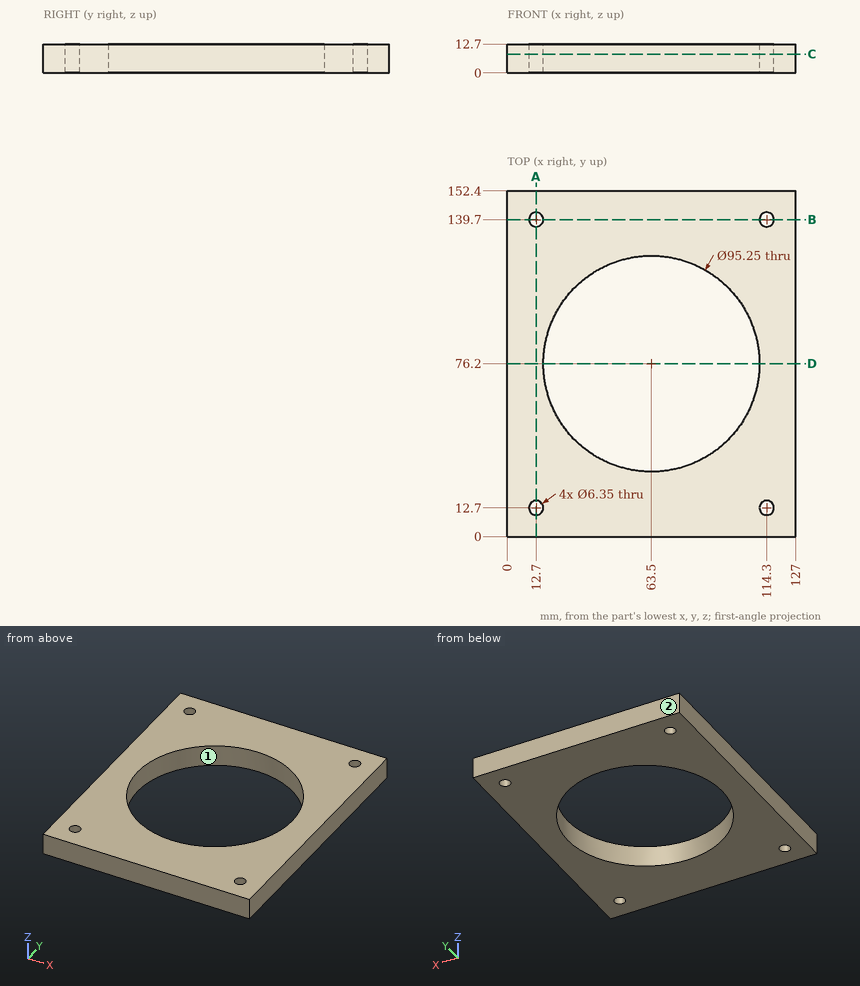
Design review of the part shown in the three views and the two pictorial views. Dimensions are in mm from the part's minimum x, y and z. Give positions to 0.01 mm unless a question says otherwise; leave off trailing zeros. Loops run counter-clockwise (first coordinate to the right, second up) from the corner with the lowest first, then second, coordinate; pieces in that order, holes last. Notation, with made-up numbers: (88, 79) -> (108, 79) arc R20 cw to (108, 87) -> close; hole circle Ø1 at (82.5, 39). An arc over 180 degrees is marked (long way). Write each question's results on one line, items separated by ' | '.
Q1. Take a section at D-D, the plane y = 76.2. Write out the cut boundary in (x, z) (3 decimals).
Reply:
outline: (0, 0) -> (15.875, 0) -> (15.875, 12.7) -> (0, 12.7) -> close; (111.125, 0) -> (127, 0) -> (127, 12.7) -> (111.125, 12.7) -> close
Q2. Take a section at B-B, the plane y = 139.7. Write out the cut boundary in (x, z) (3 decimals), plus the area to 3 significant figures.
Reply:
outline: (0, 0) -> (9.525, 0) -> (9.525, 12.7) -> (0, 12.7) -> close; (15.875, 0) -> (111.125, 0) -> (111.125, 12.7) -> (15.875, 12.7) -> close; (117.475, 0) -> (127, 0) -> (127, 12.7) -> (117.475, 12.7) -> close | area: 1,450 mm²
Q3. For pin 1 Ø4 at (x, y) = (12.7, 139.7) entering from -Z, flat-tipped, find the tip position at first contact; note if it passes through.
Reply:
pin 1: passes through
Q4. Wall thickness on L1, parallel to X at y = 12.5, z = 5.75; L2, parallel to Y at x = 12.7, z = 3.5 (3 decimals); L3, parallel to Y at x = 63.5, z = 4.5 (3 decimals): over which ranges is each line inside the solid? List them lowest first.
Reply:
L1: x = 0 to 9.53, 15.87 to 111.13, 117.47 to 127 | L2: y = 0 to 9.525, 15.875 to 136.525, 142.875 to 152.4 | L3: y = 0 to 28.575, 123.825 to 152.4
Q5. The part is to be moulded in two halves that separate along X. For the marked faces 1 and 2, say which applies: +X half, -X half, draft (parallel to the pull), parting line (faces both ways), or undercut.
Reply:
face 1: undercut | face 2: draft
Q6. Take a section at A-A, the plane x = 12.7. Write out the cut boundary in (y, z) (3 decimals).
Reply:
outline: (0, 0) -> (9.525, 0) -> (9.525, 12.7) -> (0, 12.7) -> close; (15.875, 0) -> (136.525, 0) -> (136.525, 12.7) -> (15.875, 12.7) -> close; (142.875, 0) -> (152.4, 0) -> (152.4, 12.7) -> (142.875, 12.7) -> close
Q7. Take a section at C-C, the plane z = 8.25. Write out the cut boundary in (x, y) (3 decimals), plus the area to 3 significant figures.
Reply:
outline: (0, 0) -> (127, 0) -> (127, 152.4) -> (0, 152.4) -> close; hole circle Ø6.35 at (12.7, 12.7); hole circle Ø6.35 at (12.7, 139.7); hole circle Ø95.25 at (63.5, 76.2); hole circle Ø6.35 at (114.3, 12.7); hole circle Ø6.35 at (114.3, 139.7) | area: 12,100 mm²
